For this review, take the finished solid that the model builds, in its own axes (mm). A direction names the side the tool comes from. Give positions to 0.01 mm unless a question says otherwise; leave off trailing zeros. Order: outer loops, then holes, each group sorted by start corner. A loop starts at its lowest first (then second) coordinate and runs counter-clockwise, first axis right, second up. Notation, with made-up numbers: (51, 44) - (77, 44) arc R21 ccw to (77, 70) - close; hole circle Ø2 at (-16.5, 37). An arc over 180 degrees is marked (long way). Answer as a JSON object with one key per item and string values. Group by question number.
from build123d import *

# Parameters (mm, degrees)
SKELTON_EXTRU_DEPTH = 1
SKETCH8_R           = 4
CUT_EXTRUDE1_DEPTH  = 45


with BuildPart() as part:
    # Sketch2 → skelton_extru (new body)
    with BuildSketch(Plane(origin=(0, 0, 0), x_dir=(1, 0, 0), z_dir=(0, 1, 0))):
        with BuildLine():
            Line((-4, 4), (4, 4))
            Line((4, 4), (6.7, 0.4))
            Line((6.7, 0.4), (12.5, 0.4))
            ThreePointArc((12.5, 0.4), (12.570710678, 0.429289322), (12.6, 0.5))
            Line((12.6, 0.5), (12.6, 14.5))
            ThreePointArc((12.6, 14.5), (12.863603897, 15.136396103), (13.5, 15.4))
            Line((13.5, 15.4), (15.5, 15.4))
            ThreePointArc((15.5, 15.4), (16.136396103, 15.136396103), (16.4, 14.5))
            Line((16.4, 14.5), (16.4, 0))
            Line((16.4, 0), (16.4, -14.5))
            ThreePointArc((16.4, -14.5), (16.429289322, -14.570710678), (16.5, -14.6))
            Line((16.5, -14.6), (18.5, -14.6))
            ThreePointArc((18.5, -14.6), (18.570710678, -14.570710678), (18.6, -14.5))
            Line((18.6, -14.5), (18.6, 14.5))
            ThreePointArc((18.6, 14.5), (18.863603897, 15.136396103), (19.5, 15.4))
            Line((19.5, 15.4), (21.5, 15.4))
            ThreePointArc((21.5, 15.4), (22.136396103, 15.136396103), (22.4, 14.5))
            Line((22.4, 14.5), (22.4, -14.5))
            ThreePointArc((22.4, -14.5), (22.429289322, -14.570710678), (22.5, -14.6))
            Line((22.5, -14.6), (24.5, -14.6))
            ThreePointArc((24.5, -14.6), (24.570710678, -14.570710678), (24.6, -14.5))
            Line((24.6, -14.5), (24.6, 14.5))
            ThreePointArc((24.6, 14.5), (24.863603897, 15.136396103), (25.5, 15.4))
            Line((25.5, 15.4), (27.5, 15.4))
            ThreePointArc((27.5, 15.4), (28.136396103, 15.136396103), (28.4, 14.5))
            Line((28.4, 14.5), (28.4, -14.5))
            ThreePointArc((28.4, -14.5), (28.429289322, -14.570710678), (28.5, -14.6))
            Line((28.5, -14.6), (30.5, -14.6))
            ThreePointArc((30.5, -14.6), (30.570710678, -14.570710678), (30.6, -14.5))
            Line((30.6, -14.5), (30.6, 14.5))
            ThreePointArc((30.6, 14.5), (30.863603897, 15.136396103), (31.5, 15.4))
            Line((31.5, 15.4), (33.5, 15.4))
            ThreePointArc((33.5, 15.4), (34.136396103, 15.136396103), (34.4, 14.5))
            Line((34.4, 14.5), (34.4, -14.5))
            ThreePointArc((34.4, -14.5), (34.429289322, -14.570710678), (34.5, -14.6))
            Line((34.5, -14.6), (36.5, -14.6))
            ThreePointArc((36.5, -14.6), (36.570710678, -14.570710678), (36.6, -14.5))
            Line((36.6, -14.5), (36.6, -0.5))
            ThreePointArc((36.6, -0.5), (36.863603897, 0.136396103), (37.5, 0.4))
            Line((37.5, 0.4), (47, 0.4))
            ThreePointArc((47, 0.4), (47.4, 0), (47, -0.4))
            Line((47, -0.4), (37.5, -0.4))
            ThreePointArc((37.5, -0.4), (37.429289322, -0.429289322), (37.4, -0.5))
            Line((37.4, -0.5), (37.4, -14.5))
            ThreePointArc((37.4, -14.5), (37.136396103, -15.136396103), (36.5, -15.4))
            Line((36.5, -15.4), (34.5, -15.4))
            ThreePointArc((34.5, -15.4), (33.863603897, -15.136396103), (33.6, -14.5))
            Line((33.6, -14.5), (33.6, 14.5))
            ThreePointArc((33.6, 14.5), (33.570710678, 14.570710678), (33.5, 14.6))
            Line((33.5, 14.6), (31.5, 14.6))
            ThreePointArc((31.5, 14.6), (31.429289322, 14.570710678), (31.4, 14.5))
            Line((31.4, 14.5), (31.4, -14.5))
            ThreePointArc((31.4, -14.5), (31.136396103, -15.136396103), (30.5, -15.4))
            Line((30.5, -15.4), (28.5, -15.4))
            ThreePointArc((28.5, -15.4), (27.863603897, -15.136396103), (27.6, -14.5))
            Line((27.6, -14.5), (27.6, 14.5))
            ThreePointArc((27.6, 14.5), (27.570710678, 14.570710678), (27.5, 14.6))
            Line((27.5, 14.6), (25.5, 14.6))
            ThreePointArc((25.5, 14.6), (25.429289322, 14.570710678), (25.4, 14.5))
            Line((25.4, 14.5), (25.4, -14.5))
            ThreePointArc((25.4, -14.5), (25.136396103, -15.136396103), (24.5, -15.4))
            Line((24.5, -15.4), (22.5, -15.4))
            ThreePointArc((22.5, -15.4), (21.863603897, -15.136396103), (21.6, -14.5))
            Line((21.6, -14.5), (21.6, 14.5))
            ThreePointArc((21.6, 14.5), (21.570710678, 14.570710678), (21.5, 14.6))
            Line((21.5, 14.6), (19.5, 14.6))
            ThreePointArc((19.5, 14.6), (19.429289322, 14.570710678), (19.4, 14.5))
            Line((19.4, 14.5), (19.4, -14.5))
            ThreePointArc((19.4, -14.5), (19.136396103, -15.136396103), (18.5, -15.4))
            Line((18.5, -15.4), (16.5, -15.4))
            ThreePointArc((16.5, -15.4), (15.863603897, -15.136396103), (15.6, -14.5))
            Line((15.6, -14.5), (15.6, 0))
            Line((15.6, 0), (15.6, 14.5))
            ThreePointArc((15.6, 14.5), (15.570710678, 14.570710678), (15.5, 14.6))
            Line((15.5, 14.6), (13.5, 14.6))
            ThreePointArc((13.5, 14.6), (13.429289322, 14.570710678), (13.4, 14.5))
            Line((13.4, 14.5), (13.4, 0.5))
            ThreePointArc((13.4, 0.5), (13.136396103, -0.136396103), (12.5, -0.4))
            Line((12.5, -0.4), (6.7, -0.4))
            Line((6.7, -0.4), (4, -4))
            Line((4, -4), (-4, -4))
            Line((-4, -4), (-6.7, -0.4))
            Line((-6.7, -0.4), (-12.834314575, -0.4))
            Line((-12.834314575, -0.4), (-17.076955262, -4.642640687))
            Line((-17.076955262, -4.642640687), (-31.742640687, -4.642640687))
            ThreePointArc((-31.742640687, -4.642640687), (-31.813351365, -4.671930009), (-31.842640687, -4.742640687))
            Line((-31.842640687, -4.742640687), (-31.842640687, -11.242640687))
            Line((-31.842640687, -11.242640687), (2.6, -11.242640687))
            ThreePointArc((2.6, -11.242640687), (3, -11.642640687), (2.6, -12.042640687))
            Line((2.6, -12.042640687), (-31.842640687, -12.042640687))
            Line((-31.842640687, -12.042640687), (-32.142640687, -12.042640687))
            ThreePointArc((-32.142640687, -12.042640687), (-32.496194078, -11.896194078), (-32.642640687, -11.542640687))
            Line((-32.642640687, -11.542640687), (-32.642640687, -4.742640687))
            ThreePointArc((-32.642640687, -4.742640687), (-32.37903679, -4.106244584), (-31.742640687, -3.842640687))
            Line((-31.742640687, -3.842640687), (-26.585761453, -3.842640687))
            Line((-26.585761453, -3.842640687), (-29.831514219, -0.4))
            Line((-29.831514219, -0.4), (-37.831514219, -0.4))
            ThreePointArc((-37.831514219, -0.4), (-38.231514219, 0), (-37.831514219, 0.4))
            Line((-37.831514219, 0.4), (-29.831514219, 0.4))
            Line((-29.831514219, 0.4), (-26.585761453, 3.842640687))
            Line((-26.585761453, 3.842640687), (-31.742640687, 3.842640687))
            ThreePointArc((-31.742640687, 3.842640687), (-32.37903679, 4.106244584), (-32.642640687, 4.742640687))
            Line((-32.642640687, 4.742640687), (-32.642640687, 11.542640687))
            ThreePointArc((-32.642640687, 11.542640687), (-32.496194078, 11.896194078), (-32.142640687, 12.042640687))
            Line((-32.142640687, 12.042640687), (-31.842640687, 12.042640687))
            Line((-31.842640687, 12.042640687), (2.6, 12.042640687))
            ThreePointArc((2.6, 12.042640687), (3, 11.642640687), (2.6, 11.242640687))
            Line((2.6, 11.242640687), (-31.842640687, 11.242640687))
            Line((-31.842640687, 11.242640687), (-31.842640687, 4.742640687))
            ThreePointArc((-31.842640687, 4.742640687), (-31.813351365, 4.671930009), (-31.742640687, 4.642640687))
            Line((-31.742640687, 4.642640687), (-17.076955262, 4.642640687))
            Line((-17.076955262, 4.642640687), (-12.834314575, 0.4))
            Line((-12.834314575, 0.4), (-6.7, 0.4))
            Line((-6.7, 0.4), (-4, 4))
        make_face()
        Polygon((-13.565685425, 0), (-17.408326112, -3.842640687), (-25.486266619, -3.842640687), (-29.109143003, 0), (-25.486266619, 3.842640687), (-17.408326112, 3.842640687), align=None, mode=Mode.SUBTRACT)
    extrude(amount=SKELTON_EXTRU_DEPTH)

    # Sketch3 → Revolve1 (revolve)
    with BuildSketch(Plane.XY.offset(-11.642640687), mode=Mode.PRIVATE) as revolve1_sk:
        Polygon((2.6, 0), (7.6, 0), (8.6, 4), (8.6, 50), (2.6, 50), align=None)
    revolve(revolve1_sk.sketch.rotate(Axis((2.6, 0, -11.642640687), (0, 1, 0)), 184.588565502), axis=Axis((2.6, 0, -11.642640687), (0, 1, 0)))

    # Sketch4 → Revolve2 (revolve)
    with BuildSketch(Plane(origin=(0, 0, 0), x_dir=(-1, 0, 0), z_dir=(0, 0, -1)), mode=Mode.PRIVATE) as revolve2_sk:
        Polygon((-47, 0), (-52, 0), (-53, 4), (-53, 50), (-47, 50), align=None)
    revolve(revolve2_sk.sketch.rotate(Axis((47, 0, 0), (0, 1, 0)), 184.588558424), axis=Axis((47, 0, 0), (0, 1, 0)))

    # Sketch5 → Revolve3 (revolve)
    with BuildSketch(Plane(origin=(0, 0, 0), x_dir=(-1, 0, 0), z_dir=(0, 0, -1))):
        Polygon((37.831514219, 50), (37.831514219, 0), (42.831514219, 0), (43.831514219, 4), (43.831514219, 50), align=None)
    revolve(axis=Axis((-37.831514219, 50, 0), (0, -1, 0)))

    # Sketch6 → Revolve4 (revolve)
    with BuildSketch(Plane.XY.offset(11.642640687), mode=Mode.PRIVATE) as revolve4_sk:
        Polygon((2.6, 0), (7.6, 0), (8.6, 4), (8.6, 50), (2.6, 50), align=None)
    revolve(revolve4_sk.sketch.rotate(Axis((2.6, 0, 11.642640687), (0, 1, 0)), 184.588565502), axis=Axis((2.6, 0, 11.642640687), (0, 1, 0)))

    # Sketch8 → Cut-Extrude1 (cut)
    with BuildSketch(Plane(origin=(0, 50, 0), x_dir=(1, 0, 0), z_dir=(0, 1, 0))):
        with Locations(Location((-37.831514219, 0, 0), (0, 0, 180))):
            Circle(SKETCH8_R)
        with Locations(Location((2.6, 11.642640687, 0), (0, 0, 180))):
            Circle(SKETCH8_R)
        with Locations(Location((2.6, -11.642640687, 0), (0, 0, 180))):
            Circle(SKETCH8_R)
        with Locations(Location((47, 0, 0), (0, 0, 180))):
            Circle(SKETCH8_R)
    extrude(amount=-CUT_EXTRUDE1_DEPTH, mode=Mode.SUBTRACT)


solid = part.part
1) For faces 3 (the face through (-15.46, 0.493, 1.894)), 4 (the face through (5.55, 27.82, -8.94)), list the 3-axis set-ups (+Z, -Z, +X, -X, +Y, -Y) from which the entire face can be reached by the end or side of a thin tool; tool diameter is ignored.
2) Consider section A-A (y = 32). Give the boundary of the cut face in (x, z).
3) Mouldability with a two-part tool opening along X and no side actions: class faces 1 (the face through (5.33, 0.49, -2.23)), 2 (the face through (1, 50, 7.8)) as released by +X, released by -X, zero draft, split by the parting line, or undercut.
4) Consider section B-B (x = 47). Give the boundary of the cut face in (y, z).
5) For line 1 (Z direction, x = 2.6, y = 19); line 2 (X direction, y = 14, z = 2); line 3 (Z direction, x = 1.5, y = 34), list the stretches that pass through material, from the lowest coordinate up.
6) Consider section D-D (y = 3). Give the boundary of the cut face in (x, z).
7) Consider section C-C (x = 2.6). Give the boundary of the cut face in (y, z), plus the area to 3 significant figures.
8) For pin 1 (7 mm diameter, centred on x = 2.6, z = -11.64, fed in from +Y); pin 2 (10 mm diameter, centred on x = 17, y = 25.5, fed in from -Z); pin 3 (8 mm diameter, centred on y = 32, z = 8.5, fed in from -X); pin 4 (0.5 mm diameter, centred on y = 0.5, z = 0.5, fed in from -X), all flat-tipped, find the tip position at first contact; note any pin that passes through.
Result set:
{
 "1": {"face 3": "+Y, -Y", "face 4": "+Y"},
 "2": {"outline": "circle Ø12 at (-37.83, 0); circle Ø12 at (2.6, -11.64); circle Ø12 at (2.6, 11.64); circle Ø12 at (47, 0); hole circle Ø8 at (-37.83, 0); hole circle Ø8 at (2.6, -11.64); hole circle Ø8 at (2.6, 11.64); hole circle Ø8 at (47, 0)"},
 "3": {"face 1": "undercut", "face 2": "zero draft"},
 "4": {"outline": "(0, -5) - (4, -6) - (50, -6) - (50, -4) - (5, -4) - (5, 4) - (50, 4) - (50, 6) - (4, 6) - (0, 5) - close"},
 "5": {"line 1": "z = -17.64 to -15.64, -7.64 to -5.64, 5.64 to 7.64, 15.64 to 17.64", "line 2": "x = -43.49 to -41.3, -34.37 to -32.17, 41.34 to 43.54, 50.46 to 52.66", "line 3": "z = -17.54 to -15.49, -7.8 to -5.74, 5.74 to 7.8, 15.49 to 17.54"},
 "6": {"outline": "circle Ø11.5 at (-37.83, 0); circle Ø11.5 at (2.6, -11.64); circle Ø11.5 at (2.6, 11.64); circle Ø11.5 at (47, 0)"},
 "7": {"outline": "(0, -16.64) - (4, -17.64) - (50, -17.64) - (50, -15.64) - (5, -15.64) - (5, -7.64) - (50, -7.64) - (50, -5.64) - (4, -5.64) - (0, -6.64) - close; (0, -4) - (1, -4) - (1, 4) - (0, 4) - close; (0, 6.64) - (4, 5.64) - (50, 5.64) - (50, 7.64) - (5, 7.64) - (5, 15.64) - (50, 15.64) - (50, 17.64) - (4, 17.64) - (0, 16.64) - close", "area": "480 mm2"},
 "8": {"pin 1": "stops at y = 5", "pin 2": "passes through", "pin 3": "stops at x = -41.8", "pin 4": "stops at x = -43"}
}
